```python
from build123d import *

# Parameters (mm, degrees)
F1_DEPTH    = 2
F3_DEPTH    = 10
F4_T1_DEPTH = 17.6712818196
F5_R        = 1.75
F6_DEPTH    = 2
F7_R        = 1.75
F8_DEPTH    = 2
F9_T1_DEPTH = 15
F9_T6_DEPTH = 20
F9_S7_R     = 5
F9_T8_DEPTH = 12


# Not quite as in the source:
# - a fillet or chamfer that OpenCascade refuses, or shapes differently, is made with other operations: its cross-section is extruded or revolved along the edge and cut away or added


with BuildPart() as f1:
    # F0 (on Front) → F1 (new body)
    with BuildSketch(Plane.XZ):
        with BuildLine():
            Line((-15, 0), (0, 0))
            Line((0, 0), (0, 0.1303021499))
            ThreePointArc((0, 0.1303021499), (-1.4644660941, 3.6658360558), (-5, 5.1303021499))
            Line((-5, 5.1303021499), (-29.0953893118, 5.1303021499))
            Line((-29.0953893118, 5.1303021499), (-15, 0))
        make_face()
    extrude(amount=F1_DEPTH)

    # F2 (on face) → F3 (join)
    with BuildSketch(Plane.XZ.offset(2)):
        Polygon((-23.2477805115, 5.1303021499), (-29.0953893118, 5.1303021499), (-15, 0), (0, 0), (0, 2), (-14.6473460386, 2), align=None)
    extrude(amount=F3_DEPTH)

    # F4: fillet of radius 0.2 on 1 edges, made by hand

    # F4_s2 → F4_t1 (cut)
    with BuildSketch(Plane.XZ.offset(-2.8356409098)):
        with BuildLine():
            ThreePointArc((-27.9611329479, 5.1303021499), (-28.1580944985, 4.9650317854), (-28.0295369765, 4.7423636257))
            Line((-28.0295369765, 4.7423636257), (-29.0953893118, 5.1303021499))
            Line((-29.0953893118, 5.1303021499), (-27.9611329479, 5.1303021499))
        make_face()
    extrude(amount=F4_T1_DEPTH, mode=Mode.SUBTRACT)

    # F5 (on face) → F6 (cut, through all)
    with BuildSketch(Plane(origin=(-1.07062639, 0, -2.9415218311), x_dir=(0.9396926208, 0, -0.3420201433), z_dir=(0.3420201433, 0, 0.9396926208))):
        with Locations((-20.4480432732, -7)):
            Circle(F5_R)
    extrude(amount=-F6_DEPTH, mode=Mode.SUBTRACT)

    # F7 (on face) → F8 (cut, through all)
    with BuildSketch(Plane(origin=(0, 0, 0), x_dir=(1, 0, 0), z_dir=(0, 0, -1))):
        with Locations((-6, 7)):
            Circle(F7_R)
    extrude(amount=-F8_DEPTH, mode=Mode.SUBTRACT)

    # F9: fillet of radius 2 on 1 edges, made by hand

    # F9_s2 → F9_t1 (cut)
    with BuildSketch(Plane.XZ.offset(2)):
        with BuildLine():
            ThreePointArc((0, 0), (-0.5857864376, 1.4142135624), (-2, 2))
            Line((-2, 2), (0, 2))
            Line((0, 2), (0, 0))
        make_face()
    extrude(amount=F9_T1_DEPTH, mode=Mode.SUBTRACT)


with BuildPart() as f9_tool4:
    # F9_s5 → F9_t6 (new body)
    with BuildSketch(Plane.XZ.offset(-3)):
        with BuildLine():
            ThreePointArc((0, 0), (-0.5857864376, 1.4142135624), (-2, 2))
            Line((-2, 2), (0, 2))
            Line((0, 2), (0, 0))
        make_face()
    extrude(amount=F9_T6_DEPTH)

    # F9_s7 → F9_t8 (cut, symmetric)
    with BuildSketch(Plane.XZ.offset(7)):
        with Locations((-5, 0.1303021499)):
            Circle(F9_S7_R)
    extrude(amount=F9_T8_DEPTH, both=True, mode=Mode.SUBTRACT)


with BuildPart() as f1_1:
    add(f1.part)

    # F9_t3: cut F9_tool4
    add(f9_tool4.part, mode=Mode.SUBTRACT)


solid = f1_1.part
```
Geometry check sheet. Reference: the model listing, model coordinates, mm. A direction names the side the tool comes from. Round coordinates to 2 decimals unless told otherwise and drop trailing zeros. Write each loop counter-clockwise with the first axis right and the second up, starting at its lowest first coordinate (ties: lowest second). Pieces come first, ordered by that corner, then holes. Notation, with made-up numbers: (17.5, 12) -> (74.5, 12) arc R13 ccw to (74.5, 37) -> close; hole circle Ø6 at (-24, 64.25). An arc over 180 degrees is marked (long way). Put each result on its own line as item: value.
1) Cross-section at D-D, the plane x = -15.75. Enter the section's corners in (y, z).
Recorded:
outline: (-12, 0.27) -> (0, 0.27) -> (0, 5.13) -> (-2, 5.13) -> (-2, 2.4) -> (-12, 2.4) -> close
2) Depth check by flat-ended pin: P1, Ø3, axis at x = -4.5, y = -7, coming from the -Z side; P2, Ø1.5, axis at x = -15, z = 3.5, coming from the -Y side; P3, Ø4, axis at x = -9, y = -7.5, coming from the +Z side. Enter the tip coordinate at first touch or a pass-through.
Recorded:
P1: stops at z = 0
P2: stops at y = -2
P3: stops at z = 2
3) Cross-section at C-C, the plane x = -12.25. Enter the section's corners in (y, z), plus the area to 3 significant figures.
Recorded:
outline: (-12, 0) -> (0, 0) -> (0, 5.13) -> (-2, 5.13) -> (-2, 2) -> (-12, 2) -> close
area: 30.3 mm2
4) Cross-section at A-A, the plane x = -6. Enter the section's corners in (y, z).
Recorded:
outline: (-12, 0) -> (-8.75, 0) -> (-8.75, 2) -> (-12, 2) -> close; (-5.25, 0) -> (0, 0) -> (0, 5.13) -> (-2, 5.13) -> (-2, 2) -> (-5.25, 2) -> close
5) Access from +Z, -Z, +X, -X, +Y, -Y to the whole of each face (thin tool, end or side, straight path). Record for faces 4 (the face through (-21, -1, 5.13)), 5 (the face through (-8, -7, 2)).
Recorded:
face 4: +Z, +X, -X, +Y, -Y
face 5: +Z, +X, -Y
6) Thickness scan on probe 1 along Y at (x, z) = (-6, 1.2); probe 2 along Z at (x, y) = (-12.75, -5.75); probe 3 along Y at (x, z) = (-2, 2.65). Record the ranges inside material, lowest first. Write a range as from..to.
Recorded:
probe 1: y = -12..-8.75, -5.25..0
probe 2: z = 0..2
probe 3: y = -2..0
7) Cross-section at B-B, the plane y = -8. Enter the section's corners in (x, z).
Recorded:
outline: (-28.03, 4.74) -> (-22.32, 2.66) -> (-21.64, 4.54) -> (-23.25, 5.13) -> (-27.96, 5.13) arc R0.2 ccw to start; (-19.62, 1.68) -> (-15, 0) -> (-7.44, 0) -> (-7.44, 2) -> (-14.65, 2) -> (-18.94, 3.56) -> close; (-4.56, 0) -> (0, 0) arc R2 ccw to (-2, 2) -> (-4.56, 2) -> close
8) Release check for a two-part mould opening along Y. For faces 1 (the face through (-17.932, -6.93, 3.195)), 2 (the face through (-14, -12, 1)), 3 (the face through (-21, -8.7, 3.3)) record: pulls with the +Y half, pulls with the -Y half, needs draft (parallel to the pull), parting line crosses it, or undercut.
Recorded:
face 1: needs draft
face 2: pulls with the -Y half
face 3: undercut
